Here's the drawing with two shaded views (mm, measured from the low corner). I have some questions. Coordinates: 2 decimals unless noted, no trailing zeros. Order: outer loops, then holes, each group sorted by start corner. A loop starts at its lowest first (then second) coordinate and runs counter-clockwise, first axis right, second up. Notation, with made-up numbers: (89, -5.75) -> (111, -5.75) arc R7 ccw to (111, -1.75) -> close; hole circle Ø4 at (-19.75, -17.5). An arc over 180 degrees is marked (long way). Answer as a JSON object with one key per item and string values. Group by question number.
(1) I need wall thicknesses on line 1 (Y direction, x = 92, z = 1) (1 decimal); line 2 (X direction, y = 29, z = 1.95) (1 decimal); line 3 (Y direction, x = 50, z = 1.2). Which ranges of each line are inside material? Lowest first, please.
(2) I want a section at A-A, the plane x = 26. List the corners of the cut face in (y, z) for me, plus the area to 3 significant figures.
(3) I want a section at C-C, the plane z = 0.6. State how many separate pieces and enclosed holes the cut face has, plus the area to 3 significant figures.
(4) I want a section at B-B, the plane y = 50. List the corners of the cut face in (x, z) for me, plus the area to 3 significant figures.
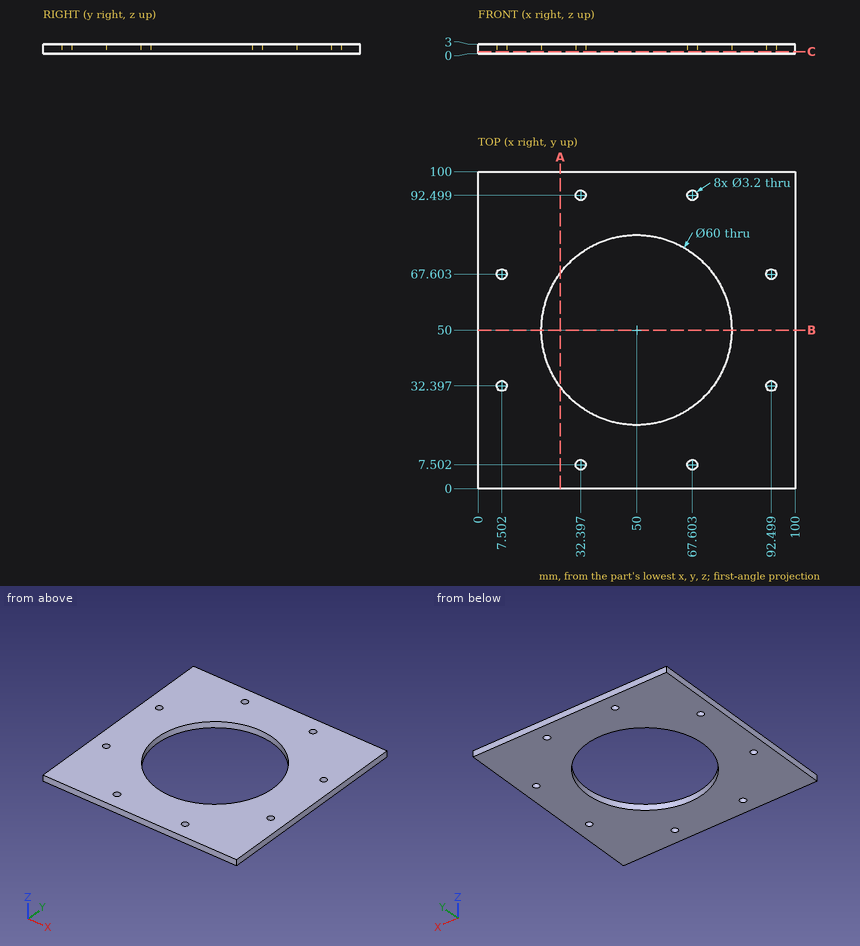
Computed values:
{
 "1": {"line 1": "y = 0 to 30.9, 33.9 to 66.1, 69.1 to 100", "line 2": "x = 0 to 28.6, 71.4 to 100", "line 3": "y = 0 to 20, 80 to 100"},
 "2": {"outline": "(0, 0) -> (32, 0) -> (32, 3) -> (0, 3) -> close; (68, 0) -> (100, 0) -> (100, 3) -> (68, 3) -> close", "area": "192 mm2"},
 "3": {"separate pieces": "1", "enclosed holes": "9", "area": "7,110 mm2"},
 "4": {"outline": "(0, 0) -> (20, 0) -> (20, 3) -> (0, 3) -> close; (80, 0) -> (100, 0) -> (100, 3) -> (80, 3) -> close", "area": "120 mm2"}
}
